```python
from build123d import *

# Parameters (mm, degrees)
ESBO_O2_R             = 2.15
CORTE_EXTRUS_O3_DEPTH = 7.8
ESBO_O3_W             = 4.788650246
ESBO_O3_H             = 2.452019704
CORTE_EXTRUS_O4_DEPTH = 3
CHANFRO1_SIZE         = 0.5
FILETE1_R             = 0.5


with BuildPart() as part:
    # Esbo_o1 → Revolu_o1 (revolve)
    with BuildSketch(Plane.XY):
        Polygon((0, 10), (0, 19.8), (2.15, 19.8), (2.15, 0), (1.55, 0), (1.55, 7.5), align=None)
    revolve(axis=Axis((0, 10, 0), (0, 1, 0)))

    # Esbo_o2 → Corte-extrus_o3 (cut)
    with BuildSketch(Plane(origin=(0, 19.8, 0), x_dir=(1, 0, 0), z_dir=(0, 1, 0))):
        Circle(ESBO_O2_R)
        with BuildLine():
            Line((-1.099159758, 1.488068488), (-0.298939494, 0.687848224))
            ThreePointArc((-0.298939494, 0.687848224), (0, 0.75), (0.298939494, 0.687848224))
            Line((0.298939494, 0.687848224), (1.099159758, 1.488068488))
            ThreePointArc((1.099159758, 1.488068488), (0, 1.85), (-1.099159758, 1.488068488))
        make_face(mode=Mode.SUBTRACT)
        with BuildLine():
            Line((-1.488068488, 1.099159758), (-0.687848224, 0.298939494))
            ThreePointArc((-0.687848224, 0.298939494), (-0.75, 0), (-0.687848224, -0.298939494))
            Line((-0.687848224, -0.298939494), (-1.488068488, -1.099159758))
            ThreePointArc((-1.488068488, -1.099159758), (-1.85, 0), (-1.488068488, 1.099159758))
        make_face(mode=Mode.SUBTRACT)
        with BuildLine():
            Line((1.099159758, -1.488068488), (0.298939494, -0.687848224))
            ThreePointArc((0.298939494, -0.687848224), (0, -0.75), (-0.298939494, -0.687848224))
            Line((-0.298939494, -0.687848224), (-1.099159758, -1.488068488))
            ThreePointArc((-1.099159758, -1.488068488), (0, -1.85), (1.099159758, -1.488068488))
        make_face(mode=Mode.SUBTRACT)
        with BuildLine():
            Line((1.488068488, 1.099159758), (0.687848224, 0.298939494))
            ThreePointArc((0.687848224, 0.298939494), (0.75, 0), (0.687848224, -0.298939494))
            Line((0.687848224, -0.298939494), (1.488068488, -1.099159758))
            ThreePointArc((1.488068488, -1.099159758), (1.85, 0), (1.488068488, 1.099159758))
        make_face(mode=Mode.SUBTRACT)
    extrude(amount=-CORTE_EXTRUS_O3_DEPTH, mode=Mode.SUBTRACT)

    # Esbo_o3 → Corte-extrus_o4 (cut)
    with BuildSketch(Plane.XZ):
        with Locations((0, 1.226009852)):
            Rectangle(ESBO_O3_W, ESBO_O3_H)
    extrude(amount=-CORTE_EXTRUS_O4_DEPTH, mode=Mode.SUBTRACT)

    # Chanfro1
    chanfro1_edges = [part.edges().sort_by_distance(p)[0] for p in [
        (0, 19.8, -0.75),
        (-0.75, 19.8, 0),
        (0.75, 19.8, 0),
        (0, 19.8, 0.75),
    ]]
    chamfer(chanfro1_edges, length=CHANFRO1_SIZE)

    # Filete1
    filete1_edges = [part.edges().sort_by_distance(p)[0] for p in [
        (0, 19.8, -1.85),
        (-1.85, 19.8, 0),
        (1.85, 19.8, 0),
        (0, 19.8, 1.85),
    ]]
    fillet(filete1_edges, radius=FILETE1_R)


solid = part.part
```
Source: CAD feature listing. Evaluate the final solid. Frame: model axes, mm. A direction names the side the tool comes from. Coordinates: 2 decimals unless noted, no trailing zeros. Loops run counter-clockwise (first coordinate to the right, second up) from the corner with the lowest first, then second, coordinate; pieces in that order, holes last. Notation, with made-up numbers: M -38.5,88 L -12.5,88 A24 cw -12.5,105 Z; hole C -26,-13.5 d6. An arc over 180 degrees is marked long. Put each result on its own line as item: value. Start each with the question number.
1) Contact query for flat-ended pins moving along their axis: pin 1 Ø0.7 at (x, y) = (-2, 1.5) entering from +Z; pin 2 Ø2.5 at (x, z) = (0, 1.5) entering from -Y; pin 3 Ø1 at (y, z) = (13, 1) entering from +X. Output: stop coordinate, or through.
2) Cut plane A-A on y = 11. Return the cut outline in (x, z).
3) Cut plane B-B on y = 8.25. Return the cut outline in (x, z) (3 decimals), then the cut area to 3 significant figures.
4) Reachability of faces 1 (the face through (0, 3, 1.8)), 2 (the face through (0.7, 15.95, 1.09)), 3 (the face through (-0.202, 4.636, -1.537)), 4 (the face through (-0.02, 15.7, 1.85)) from +Z, -Z, +X, -X, +Y, -Y: full face, straight path, thin tool, end or side. Return the list, or none.
5) Pull-direction query (Z, two-part tool) for faces 5 (the face through (1.09, 15.95, -0.7)), 6 (the face through (0.02, 15.7, -1.85)), 7 (the face through (-1.85, 15.7, 0.02)); classes: pulls with the +Z half, pulls with the -Z half, needs draft (parallel to the pull), parting line crosses it, or undercut.
6) Ray query, L1, parallel to X at y = 5.5, z = -0.1; L2, parallel to Z at x = 0, y = 2.75. Return the intervals inside material, ascending. Write a range as from..to.
The answers:
1. pin 1: stops at z = 0
1. pin 2: stops at y = 3
1. pin 3: stops at x = 1.78
2. outline: C 0,0 d4.3
3. outline: C 0,0 d4.3; hole C 0,0 d2.17
3. area: 10.8 mm²
4. face 1: +Z, +X, -X, -Y
4. face 2: +Y
4. face 3: -Y
4. face 4: +Z, +Y
5. face 5: undercut
5. face 6: pulls with the -Z half
5. face 7: parting line crosses it
6. L1: x = -2.15..-1.55, 1.55..2.15
6. L2: z = -2.15..-1.55
